The model under review builds one solid part; all positions refer to its coordinate system, in mm. Face numbers are marked on the shaded views. A direction names the side the tool comes from. Coordinates: 2 decimals unless noted, no trailing zeros. Order: outer loops, then holes, each group sorted by start corner. A loop starts at its lowest first (then second) coordinate and runs counter-clockwise, first axis right, second up. Notation, with made-up numbers: M 26.25,72 L 74.25,72 A10 ccw 74.25,86 Z; hole C 80,-28.75 d7. An arc over 180 degrees is marked long. Answer in a Markdown table with one row per item.
from build123d import *

# Parameters (mm, degrees)
BOSS_EXTRUDE1_DEPTH = 40


with BuildPart() as part:
    # Sketch1 → Boss-Extrude1 (new body)
    with BuildSketch(Plane.XY):
        with BuildLine():
            Line((0, 12), (10, 12))
            Line((10, 12), (10, 27))
            Line((10, 27), (12, 27))
            Line((12, 27), (12, 10))
            Line((12, 10), (0, 10))
            ThreePointArc((0, 10), (-10, 0), (0, -10))
            Line((0, -10), (12, -10))
            Line((12, -10), (12, -27))
            Line((12, -27), (10, -27))
            Line((10, -27), (10, -12))
            Line((10, -12), (0, -12))
            ThreePointArc((0, -12), (-12, 0), (0, 12))
        make_face()
    extrude(amount=BOSS_EXTRUDE1_DEPTH)


solid = part.part
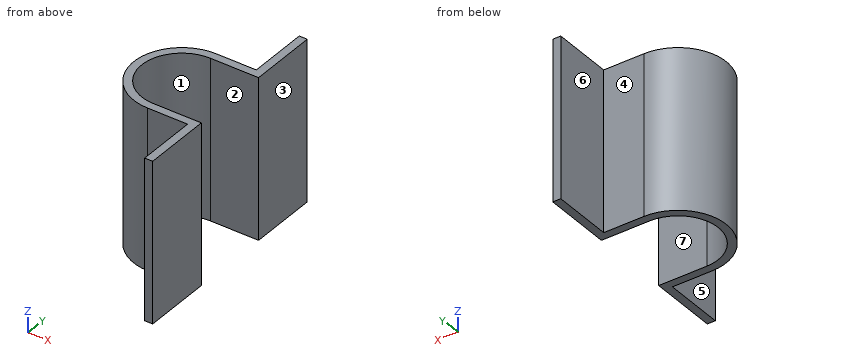
(1) Machinability: for the marked faces 5, 6 and 7, which of the approach directions +Z, -Z, +X, -X, +Y, -Y give a long, thin tool a straight path to every point of the face, cutting with its end or side? Answer none if there is none.
Report:
| item | result |
|---|---|
| face 5 | +Z, -Z, -X, -Y |
| face 6 | +Z, -Z, -X, +Y |
| face 7 | +Z, -Z, +X |
(2) Insertion check: P1, Ø16.5, axis at y = 16, z = 27, coming from the -X side; P2, Ø5, axis at x = 2, z = 8, coming from the +Y side; P3, Ø10, axis at y = -17.5, z = 16, coming from the -X side. Each pin has a flat end and moves straight along its axis. Give the tip position at first contact, or say it passes through.
Report:
| item | result |
|---|---|
| P1 | x = -9.16 |
| P2 | y = 12 |
| P3 | x = 10 |
(3) Take a section at B-B (z = 38.5). Write out the cut boundary in (x, y).
Report:
| item | result |
|---|---|
| outline | M 0,-12 L 10,-12 L 10,-27 L 12,-27 L 12,-10 L 0,-10 A10 cw 0,10 L 12,10 L 12,27 L 10,27 L 10,12 L 0,12 A12 ccw Z |
(4) Take a section at D-D (y = 9). Write out the cut boundary in (x, z).
Report:
| item | result |
|---|---|
| outline | M -7.94,0 L -4.36,0 L -4.36,40 L -7.94,40 Z |
(5) To check wall thickness, follow line 1 (Y direction, x = 11.25, z = 32.5); line 2 (Y direction, x = 2.5, z = 28.5); line 3 (X direction, y = 15, z = 24.5). State the ranges of each line that lie inside material, in increasing order. Write a range as [from, to].
Report:
| item | result |
|---|---|
| line 1 | [-27, -10], [10, 27] |
| line 2 | [-12, -10], [10, 12] |
| line 3 | [10, 12] |
(6) The part is to be moulded in two halves that separate along Y. For the marked faces 1, 2, 3 and 4, say which applies: +Y half, -Y half, draft (parallel to the pull), parting line (faces both ways), or undercut.
Report:
| item | result |
|---|---|
| face 1 | undercut |
| face 2 | undercut |
| face 3 | draft |
| face 4 | +Y half |
(7) Take a section at C-C (y = 0). Write out the cut boundary in (x, z).
Report:
| item | result |
|---|---|
| outline | M -12,0 L -10,0 L -10,40 L -12,40 Z |
(8) Take a section at A-A (x = 5). Write out the cut boundary in (y, z), then the cut area to 3 significant figures.
Report:
| item | result |
|---|---|
| outline | M -12,0 L -10,0 L -10,40 L -12,40 Z; M 10,0 L 12,0 L 12,40 L 10,40 Z |
| area | 160 mm^2 |
